CAD build for the part. Positions are in the model's coordinates, mm. A direction names the side the tool comes from. Round coordinates to 2 decimals unless told otherwise and drop trailing zeros. Loops run counter-clockwise (first coordinate to the right, second up) from the corner with the lowest first, then second, coordinate; pieces in that order, holes last. Notation, with made-up numbers: (4, -10) - (62, -10) arc R31 ccw to (62, 23) - close; hole circle Ø1 at (-26, 38.5). An arc over 180 degrees is marked (long way). One line per question, with ' | ' between items.
Autodesk Inventor part; units mm, degrees
ref_plane "Plan de courroie" through (0, 105.5, 11) normal (0, 0, 1) x (1, 0, 0)
ref_plane "XZ Plane" through (0, 0, 0) normal (0, 1, 0) x (-1, 0, 0)
ref_plane "XY Plane" through (0, 0, 0) normal (0, 0, 1) x (1, 0, 0)
sketch "Esquisse principale" plane through (0, 0, 0) normal (1, 0, 0) x (0, 1, 0)
  line L0 (0, 22) -> (116.5, 22)
  line L1 (116.5, 22) -> (116.5, 18.6115)
  line L2 (116.5, 18.6115) -> (105.5, 15.2484)
  line L3 (105.5, 15.2484) -> (105.5, 6.7516)
  line L4 (105.5, 6.7516) -> (116.5, 3.3885)
  line L5 (116.5, 3.3885) -> (116.5, 0)
  line L6 (116.5, 0) -> (0, 0)
  line L7 (114.5, 18) -> (114.5, 4) construction
  line L8 (105.5, 11) -> (114.5, 11) construction
  line L9 (116.5, 18.6115) -> (116.5, 3.3885)
  line L10 (0, -4.4) -> (0, 26.4)
  line L11 (0, 0) -> (0, 22)
  dimension "d0" = 14
  dimension "d1" = 34
  dimension "d2" = 2
  dimension "d6" = 22
  dimension "d21" = 229
  dimension "d25" = 11
  dimension "d27" = 11
ref_plane "Plan de courroie" through (0, 105.5, 11) normal (0, 0, 1) x (1, 0, 0)
revolve "Corps" add sketch "Esquisse principale" angle 360 about axis through (0, 0, -10) along (0, 0, 1)
revolve "Bord" cut sketch "Esquisse principale" angle 360 about axis through (0, 0, -10) along (0, 0, 1) contours L9 L4 L3 L2
fillet "Congé externe" [suppressed]
fillet "Congé interne" [suppressed]
sketch "Esquisse4" plane through (0, 0, 0) normal (1, 0, 0) x (0, 1, 0)
  line L0 (0, -20.2967) -> (0, 37.5815)
  line L1 (12.5, 32.25) -> (12.5, -12.25)
  line L2 (12.5, -12.25) -> (36.75, -12.25)
  line L3 (12.5, 32.25) -> (42.75, 32.25)
  line L4 (42.75, 32.25) -> (36.75, -12.25)
  line L5 (-116.5, 0) -> (116.5, 0)
  line L6 (12.5, 32.25) -> (0, 32.25)
  line L7 (12.5, -12.25) -> (0, -12.25)
  line L8 (0, -12.25) -> (0, 32.25)
  point P0 (0, 0)
  point P1 (0, 0)
  point P2 (12.5, 0)
  dimension "d48" = 12.5
  dimension "d49" = 73.5
  dimension "d50" = 85.5
  dimension "d51" = 44.5
  dimension "d52" = 12.25
revolve "Révolution3" cut sketch "Esquisse4" angle 360 about axis through (0, 0, -20.2967) along (0, 0, 1) contours L0 L6 L1 L5 | L1 L5 L4 L2 | L1 L3 L4 L5
sketch "Esquisse5" plane through (0, 0, 22) normal (0, 0, 1) x (1, 0, 0)
  line L0 (0, 0) -> (97.3173, 0)
  line L1 (0, 0) -> (-92.8604, 0)
  line L2 (0, 0) -> (0, -102.459)
  circle A0 centre (0, 0) radius 40.9
  point P0 (0, 0)
  point P1 (0, -40.9)
  point P2 (-40.9051, 0)
  point P3 (40.9, 0)
  dimension "d68" = 81.8
hole "Perçage3" at (0, -40.9, 22) at (-40.9051, 0, 22) at (40.9, 0, 22) direction (0, 0, -1) diameter 10.106 depth 15 tip angle 118
equation "\"d0\" = da_Bw"
equation "\"d1\" = da_Alfa"
equation "\"d2\" = da_c"
equation "\"d21\" = da_Dw"
equation "\"d25\" = da_Hd"
equation "\"d27\" = da_Se"
equation "\"da_r1\" = 0"
equation "\"da_r2\" = 0"
equation "\"d5\" = da_Se"
equation "\"da_Bw\" = 14"
equation "\"da_Alfa\" = 34deg"
equation "\"da_c\" = 2"
equation "\"da_Dw\" = 229"
equation "\"da_Hd\" = 11"
equation "\"da_Se\" = 11"
equation "\"da_Sg\" = 12"
properties part number "Poulie à gorge1" material "Steel"
(1) Cut at A-A, the plane z = 12. Write the cut outline in (x, y), then the cut area to 3 significant figures.
Results found:
outline: circle Ø211 at (0, 0); hole (-39.72, -4.91) arc R40.02 ccw to (-4.91, -39.72) arc R5.05 ccw (long way) to (4.91, -39.72) arc R40.02 ccw to (39.72, -4.91) arc R5.05 ccw (long way) to (39.72, 4.91) arc R40.02 ccw to (-39.72, 4.91) arc R5.05 ccw (long way) to start | area: 29,800 mm²
(2) Two-plate mould, pull along X, no slides. Class faces 1 (the face through (15.032, 36.254, 6.265)), 2 (the face through (-103.66, -23.02, 6.54)), 3 (the face through (-28, -28, 0)): released by +X, released by -X, zero draft, split by the parting line, or undercut.
Results found:
face 1: undercut | face 2: split by the parting line | face 3: zero draft
(3) Probe L1, parallel to X at y = 16, z = 10.25; L2, parallel to X at y = 0, z = 14; L3, parallel to Y at x = -15.5, z = 8.5. List the from-to ranges inside material, lowest first.
Results found:
L1: x = -104.28 to -36.42, 36.42 to 104.28 | L2: x = -105.5 to -45.96, 45.95 to 105.5 | L3: y = -104.36 to -36.38, 36.38 to 104.36
(4) Drop flat-ended pins along their axis: P1, Ø12, axis at x = 47, z = 8, coming from the +Y side; P2, Ø4, axis at x = 65, z = 19, coming from the +Y side; P3, Ø4, axis at x = 69, z = 18.5, coming from the -Y side. Give the stop position or say it passes through.
Results found:
P1: stops at y = 108.21 | P2: stops at y = 98 | P3: stops at y = -95.3
(5) Tool access for faces 4 (the face through (0.14, -45.95, 14.4)), 5 (the face through (-31.896, 101.285, 15.459)), 6 (the face through (-70.89, -92.45, 20.28)): list every direction of +Z, -Z, +X, -X, +Y, -Y with a clear straight run to the whole face (end or side of a thin tool).
Results found:
face 4: +Z | face 5: none | face 6: +Z, -Z
